Input: part model. Units: mm. Frame: model coordinates. A direction names the side the tool comes from. Give positions to 0.01 mm unless a question says otherwise; leave off trailing zeros. Loops run counter-clockwise (first coordinate to the right, second up) from the corner with the lowest first, then second, coordinate; pieces in that order, holes last. Notation, with made-up numbers: (14.25, -27.5) - (36.25, -27.5) arc R13 ccw to (36.25, -3.5) - close; hole circle Ø2 at (-38, -16). An arc over 180 degrees is marked (long way). One line per item, written item: value.
from build123d import *

# Parameters (mm, degrees)
F1_DEPTH      = 5
F3_DEPTH      = 1.5
F3_DEPTH_BACK = 1.5
F5_DEPTH      = 6.23198
F6_DEPTH      = 3.21356


with BuildPart() as f1:
    # F0 (on Top) → F1 (new body)
    with BuildSketch(Plane.XY):
        Polygon((1.5, 2), (-1.5, 2), (-1.5, -2), (-1.282606, -2), (1.282606, -2), (1.5, -2), align=None)
    extrude(amount=F1_DEPTH)

    # F2 (on Right) → F3 (join, two sides)
    with BuildSketch(Plane.YZ) as f3_sk:
        Polygon((-2, 5), (2, 5), (-2, 6.433511), align=None)
    extrude(amount=F3_DEPTH)
    extrude(f3_sk.sketch, amount=-F3_DEPTH_BACK)

    # F4 (on Front) → F5 (cut)
    with BuildSketch(Plane.XZ):
        with BuildLine():
            Line((1.096531, 0), (1.096531, 4.195458))
            ThreePointArc((1.096531, 4.195458), (0, 5.29199), (-1.096531, 4.195458))
            Line((-1.096531, 4.195458), (-1.096531, 0))
            Line((-1.096531, 0), (1.096531, 0))
        make_face()
    extrude(amount=F5_DEPTH, mode=Mode.SUBTRACT)

    # F0 (on Top) → F6 (join)
    with BuildSketch(Plane.XY):
        Polygon((-1.282606, -2), (-1.5, -2), (-1.5, -2.462873), (1.5, -2.462873), (1.5, -2), (1.282606, -2), (1.282606, -2.277132), (-1.282606, -2.277132), align=None)
    extrude(amount=F6_DEPTH)


solid = f1.part
Item 1: Section C-C, the plane x = 0. Output: boundary loops of the cut face in (y, z).
Verdict:
outline: (-2.46, 0) - (-2.28, 0) - (-2.28, 3.21) - (-2.46, 3.21) - close; (-2, 5.29) - (0, 5.29) - (0, 0) - (2, 0) - (2, 5) - (-2, 6.43) - close
Item 2: Section D-D, the plane y = -1.05. Output: boundary loops of the cut face in (x, z).
Verdict:
outline: (-1.5, 0) - (-1.1, 0) - (-1.1, 4.2) arc R1.1 cw to (1.1, 4.2) - (1.1, 0) - (1.5, 0) - (1.5, 6.09) - (-1.5, 6.09) - close
Item 3: Pin query (flat end, axial travel): P1, Ø0.5, axis at x = -0.5, y = -2.5, coming from the +Z side. Return the tip coordinate at first contact, or that it passes through.
Verdict:
P1: stops at z = 3.21
Item 4: Access query for faces 1 (the face through (0.02, -0.99, 5.29)), 2 (the face through (1, -2, 5)), 3 (the face through (-1.097, -1, 2)), 4 (the face through (0, -2.277, 2)). Directions: +Z, -Z, +X, -X, +Y, -Y. A direction counts if a zero-diameter tool reaches every point of the face in a straight line with its end or side. Return the directions, or none.
Verdict:
face 1: -Z, -Y
face 2: +Z
face 3: -Z
face 4: +Z, -Z
Item 5: Section B-B, the plane z = 2. Output: boundary loops of the cut face in (x, y), and give its area (3 significant figures).
Verdict:
outline: (-1.5, -2.46) - (1.5, -2.46) - (1.5, 2) - (-1.5, 2) - close; hole (-1.28, -2.28) - (1.28, -2.28) - (1.28, -2) - (1.1, -2) - (1.1, 0) - (-1.1, 0) - (-1.1, -2) - (-1.28, -2) - close
area: 8.29 mm^2
Item 6: Section A-A, the plane x = -1.2. Output: boundary loops of the cut face in (y, z), and give its area (3 significant figures).
Verdict:
outline: (-2.46, 0) - (-2.28, 0) - (-2.28, 3.21) - (-2.46, 3.21) - close; (-2, 0) - (2, 0) - (2, 5) - (-2, 6.43) - close
area: 23.5 mm^2
Item 7: Draft query along X for faces 5 (the face through (0, 0, 3)), 6 (the face through (1.5, 0, 2)), 7 (the face through (0.021, 0.028, 5.707)). Return one class per face: pulls with the +X half, pulls with the -X half, needs draft (parallel to the pull), parting line crosses it, or undercut.
Verdict:
face 5: undercut
face 6: pulls with the +X half
face 7: needs draft
Item 8: Material intervals for L1, parallel to Y at x = -0.35, z = 3; L2, parallel to X at y = -0.25, z = 2.5; L3, parallel to Y at x = -0.65, z = 4.75, sorted ascending.
Verdict:
L1: y = -2.46 to -2.28, 0 to 2
L2: x = -1.5 to -1.1, 1.1 to 1.5
L3: y = 0 to 2
